Read the model definition and answer for the solid it produces. Units are mm, in the model's axes. Coordinates: 2 decimals unless noted, no trailing zeros. Loops run counter-clockwise (first coordinate to the right, second up) from the corner with the lowest first, then second, coordinate; pieces in that order, holes last. Notation, with made-up numbers: M -27,-27.75 L -23,-27.75 A14 cw -23,-8.75 Z; hole C 23,-29 d8. An arc over 180 degrees is marked long. Put each result on its own line as item: value.
from build123d import *

# Parameters (mm, degrees)
F1_DEPTH    = 2
F0_W        = 2
F0_H        = 5
F2_DEPTH    = 6
F3_W        = 4
F3_H        = 5
F4_DEPTH    = 1.2
F5_W        = 4
F5_H        = 5
F6_DEPTH    = 1.2
F7_T1_DEPTH = 25.5734639037


# Not quite as in the source:
# - a fillet or chamfer that OpenCascade refuses, or shapes differently, is made with other operations: its cross-section is extruded or revolved along the edge and cut away or added


with BuildPart() as f1:
    # F0 (on Front) → F1 (new body)
    with BuildSketch(Plane.XZ):
        with BuildLine():
            ThreePointArc((86, 16), (80.1421356237, 30.1421356237), (66, 36))
            Line((66, 36), (-66, 36))
            ThreePointArc((-66, 36), (-80.1421356237, 30.1421356237), (-86, 16))
            Line((-86, 16), (-86, 2.5))
            Line((-86, 2.5), (-84, 2.5))
            Line((-84, 2.5), (-84, -2.5))
            Line((-84, -2.5), (-86, -2.5))
            Line((-86, -2.5), (-86, -16))
            ThreePointArc((-86, -16), (-80.1421356237, -30.1421356237), (-66, -36))
            Line((-66, -36), (66, -36))
            ThreePointArc((66, -36), (80.1421356237, -30.1421356237), (86, -16))
            Line((86, -16), (86, -2.5))
            Line((86, -2.5), (84, -2.5))
            Line((84, -2.5), (84, 2.5))
            Line((84, 2.5), (86, 2.5))
            Line((86, 2.5), (86, 16))
        make_face()
    extrude(amount=F1_DEPTH)

    # F0 (on Front) → F2 (join)
    with BuildSketch(Plane.XZ):
        with Locations((85, 0)):
            Rectangle(F0_W, F0_H)
        with Locations((-85, 0)):
            Rectangle(F0_W, F0_H)
    extrude(amount=F2_DEPTH)

    # F3 (on face) → F4 (join)
    with BuildSketch(Plane(origin=(-86, 0, 0), x_dir=(0, -1, 0), z_dir=(-1, 0, 0))):
        with Locations((4, 0)):
            Rectangle(F3_W, F3_H)
    extrude(amount=F4_DEPTH)

    # F5 (on face) → F6 (join)
    with BuildSketch(Plane.YZ.offset(86)):
        with Locations((-4, 0)):
            Rectangle(F5_W, F5_H)
    extrude(amount=F6_DEPTH)

    # F7: chamfer of 4 on 2 edges, made by hand

    # F7_s2 → F7_t1 (cut)
    with BuildSketch(Plane.XY.offset(-12.7867319519)):
        Polygon((83.2, -6), (87.2, -2), (87.2, -6), align=None)
        Polygon((-83.2, -6), (-87.2, -2), (-87.2, -6), align=None)
    extrude(amount=F7_T1_DEPTH, mode=Mode.SUBTRACT)


solid = f1.part
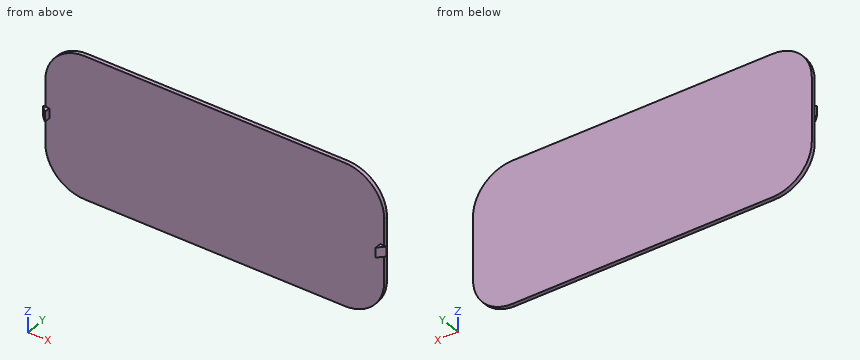
1) Given pin 1 Ø1 at (x, y) = (11, -3) entering from -Z; pin 2 Ø2.5 at (x, y) = (-85, -4) entering from -Z; pin 3 Ø1 at (x, y) = (-85, -3.5) entering from +Z; pin 4 Ø0.6 at (x, z) = (87, 0.5) entering from +Y, each flat-ended and moving along its own axis, determine where each tip first touches the part or whether it passes through.
Answer list:
pin 1: passes through
pin 2: stops at z = -2.5
pin 3: stops at z = 2.5
pin 4: stops at y = -2
2) Find section B-B, the plane z = -4.5. Write down the section's boundary in (x, y), plus the area to 3 significant figures.
Answer list:
outline: M -86,-2 L 86,-2 L 86,0 L -86,0 Z
area: 344 mm^2
3) Find section A-A, the plane x = 32.5. Write down the section's boundary in (y, z), plus the area to 3 significant figures.
Answer list:
outline: M -2,-36 L 0,-36 L 0,36 L -2,36 Z
area: 144 mm^2
4) Straight lines are drawn through the part: line 1 (Y direction, x = 77, z = 19.5); line 2 (X direction, y = -1.15, z = -16); line 3 (Z direction, x = -67, y = -1.2). For each, find the intervals that lie inside material, in ascending order. Write a range as [from, to].
Answer list:
line 1: y = [-2, 0]
line 2: x = [-86, 86]
line 3: z = [-35.97, 35.97]
